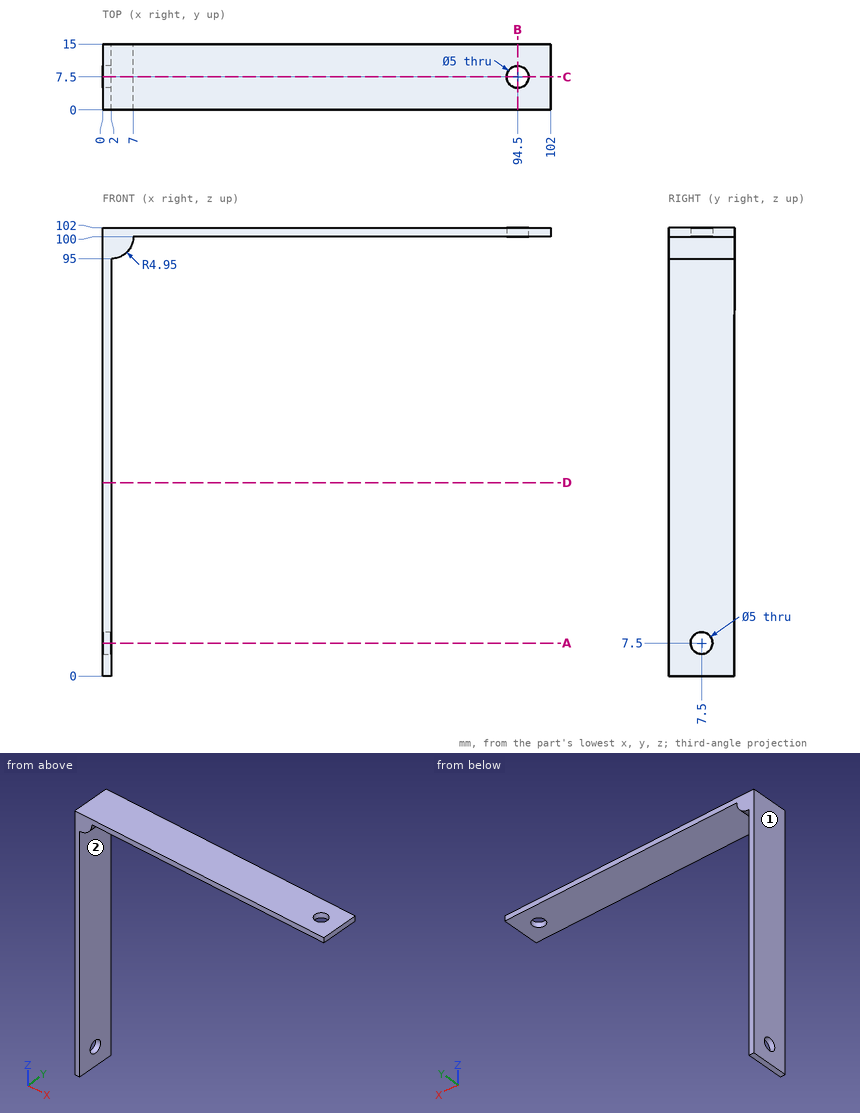
Check sheet for the drawn part. Datum: minimum x, y, z corner. Units: mm. A direction names the side the tool comes from. Give positions to 0.01 mm unless a question says otherwise; leave off trailing zeros. Order: outer loops, then holes, each group sorted by start corner. A loop starts at its lowest first (then second) coordinate and runs counter-clockwise, first axis right, second up. Notation, with made-up numbers: (-23.75, -7) -> (17.25, -7) arc R15 ccw to (17.25, 5) -> close; hole circle Ø3 at (27, -26). An arc over 180 degrees is marked (long way). One line per item, written item: value.
(1) Sectioned sample at D-D on z = 44. Record the cut outline in (x, y), then the cut area to 3 significant figures.
Final values:
outline: (0, 0) -> (2, 0) -> (2, 15) -> (0, 15) -> close
area: 30.0 mm^2
(2) Gauge pin test, flat ends, axial feed: pin 1 (6 mm diameter, centred on x = 94.5, y = 7.5, fed in from -Z); pin 2 (4.5 mm diameter, centred on y = 7.5, z = 7.5, fed in from -X); pin 3 (7.5 mm diameter, centred on y = 4, z = 37.5, fed in from +X). Record the tip position at first contact, or that the pin passes through.
Final values:
pin 1: z = 100
pin 2: through
pin 3: x = 2
(3) Scan lines: line 1 along Z through (x, y) = (96, 12); line 2 along X through (y, z) = (7.25, 84.5); line 3 along Y through (x, z) = (1, 7). Record each from-to range of solid material in increasing order. Write a range as [from, to].
Final values:
line 1: [100, 102]
line 2: [0, 2]
line 3: [0, 5.05], [9.95, 15]
(4) Sectioned sample at A-A on z = 7.5. Record the cut outline in (x, y).
Final values:
outline: (0, 0) -> (2, 0) -> (2, 5) -> (0, 5) -> close; (0, 10) -> (2, 10) -> (2, 15) -> (0, 15) -> close
(5) Tool access check on the marked faces 1 and 2. Record the directions out of +Z, -Z, +X, -X, +Y, -Y that give a thin tool (end or side, any length) a straight path to the whole face; none if there is none.
Final values:
face 1: +Z, -Z, -X, +Y, -Y
face 2: -Z, +X, +Y, -Y
(6) Sectioned sample at C-C on y = 7.5. Record the cut outline in (x, z).
Final values:
outline: (0, 0) -> (2, 0) -> (2, 5) -> (0, 5) -> close; (0, 10) -> (2, 10) -> (2, 95) -> (2.05, 95) arc R4.95 ccw to (7, 99.95) -> (7, 100) -> (92, 100) -> (92, 102) -> (0, 102) -> close; (97, 100) -> (102, 100) -> (102, 102) -> (97, 102) -> close
(7) Sectioned sample at B-B on x = 94.5. Record the cut outline in (y, z), then the cut area to 3 significant figures.
Final values:
outline: (0, 100) -> (5, 100) -> (5, 102) -> (0, 102) -> close; (10, 100) -> (15, 100) -> (15, 102) -> (10, 102) -> close
area: 20.0 mm^2
